Read the model definition and answer for the solid it produces. Units are mm, in the model's axes. Face numbers are marked on the shaded views. Give positions to 0.01 mm unless a question says otherwise; leave off trailing zeros. Loops run counter-clockwise (first coordinate to the right, second up) from the corner with the lowest first, then second, coordinate; pieces in that order, holes last.
(1) Find section B-B, the plane z = -4. Write down the section's boundary in (x, y) (3 decimals), then the cut area to 3 significant figures.
(2) Determine the mould class of the marked faces 1, 2, 3 and 4 for opening direction X: pulls with the +X half, pulls with the -X half, needs draft (parallel to the pull), parting line crosses it, or undercut.
(3) Find section A-A, the plane y = 0. Write down the section's boundary in (x, z), then the cut area to 3 significant figures.
(4) Straight lines are drawn through the part: probe 1 along Y at (x, z) = (-2.75, -0.3); probe 2 along X at (y, z) = (3.5, -1.15); probe 3 along X at (y, z) = (3.25, -0.9). For each, find the intervals that lie inside material, in ascending order.
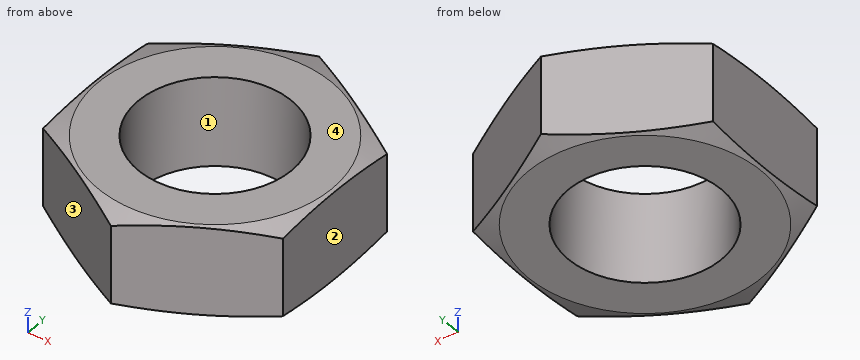
```python
from build123d import *

# Parameters (mm, degrees)
SKETCH_3_OUTSIDE_W  = 20.708
SKETCH_3_OUTSIDE_H  = 20.708
CUT_EXTRUDE_2_DEPTH = 4.7


with BuildPart() as part:
    # Эскиз2 → Повернуть1 (revolve)
    with BuildSketch(Plane(origin=(0, 0, 0), x_dir=(0, 0, -1), z_dir=(1, 0, 0)), mode=Mode.PRIVATE) as revolve_1_sk:
        Polygon((0, 4), (0, 6.1), (0.3, 7.25), (4.4, 7.25), (4.7, 6.1), (4.7, 4), align=None)
    revolve(revolve_1_sk.sketch.rotate(Axis((0, 0, 0), (0, 0, -1)), 90), axis=Axis((0, 0, 0), (0, 0, -1)))

    # Эскиз3 outside → Вытянуть2 (cut)
    with BuildSketch(Plane.XY):
        Rectangle(SKETCH_3_OUTSIDE_W, SKETCH_3_OUTSIDE_H)
        Polygon((0, 7.25), (-6.278684177, 3.625), (-6.278684177, -3.625), (0, -7.25), (6.278684177, -3.625), (6.278684177, 3.625), align=None, mode=Mode.SUBTRACT)
    extrude(amount=-CUT_EXTRUDE_2_DEPTH, mode=Mode.SUBTRACT)


solid = part.part
```
Entries:
1. outline: (-6.279, -3.625) - (0, -7.25) - (6.279, -3.625) - (6.279, 3.625) - (0, 7.25) - (-6.279, 3.625) - close; hole circle Ø8 at (0, 0)
1. area: 86.3 mm2
2. face 1: undercut
2. face 2: pulls with the +X half
2. face 3: pulls with the -X half
2. face 4: needs draft
3. outline: (-6.28, -4.65) - (-6.1, -4.7) - (-4, -4.7) - (-4, 0) - (-6.1, 0) - (-6.28, -0.05) - close; (4, -4.7) - (6.1, -4.7) - (6.28, -4.65) - (6.28, -0.05) - (6.1, 0) - (4, 0) - close
3. area: 21.4 mm2
4. probe 1: y = -5.66 to -2.9, 2.9 to 5.66
4. probe 2: x = -6.28 to -1.94, 1.94 to 6.28
4. probe 3: x = -6.28 to -2.33, 2.33 to 6.28
